Build history of the part. All positions in model axes, mm. A direction names the side the tool comes from. Give positions to 0.01 mm unless a question says otherwise; leave off trailing zeros. One line per item, written item: value.
```python
from build123d import *

# Parameters (mm, degrees)
F2_R     = 2.54
F3_R     = 1
F4_W     = 19.7092390154
F4_H     = 15.7092064619
F5_DEPTH = 22.4


with BuildPart() as f1:
    # F0 (on Front) → F1 (revolve)
    with BuildSketch(Plane.XZ):
        with BuildLine():
            Line((0, 130), (0, 0))
            Line((0, 0), (17.5, 0))
            add(Edge.make_bspline(
                [(17.5, 130), (22.5, 119.6596379665), (24.4853151406, 100.3614181833), (17.1932288242, 80.5399245506), (13.9866485718, 64.883493419), (17.1932288242, 49.9643932696), (24.4853151406, 27.3672993347), (22.5, 16.2580761236), (17.5, 0)],
                knots=[0, 0, 0, 0, 0.1975961429, 0.3602784274, 0.5, 0.6397215726, 0.8024038571, 1, 1, 1, 1], degree=3))
            add(Edge.make_bspline(
                [(3, 205), (1.2158900885, 130), (5.5774394423, 104.8566326499), (17.5, 130)],
                knots=[0, 0, 0, 0, 76.3888080808, 76.3888080808, 76.3888080808, 76.3888080808], degree=3))
            Line((3, 205), (0, 205))
            Line((0, 205), (0, 130))
        make_face()
        Polygon((0, 210), (0, 205), (3, 205), (5, 205), (5, 210), align=None)
    revolve(axis=Axis((0, 0, 65), (0, 0, 1)))

    # F2
    f2_edges = [f1.edges().sort_by_distance(p)[0] for p in [
        (-17.5, 0, 0),
    ]]
    fillet(f2_edges, radius=F2_R)

    # F3
    f3_edges = [f1.edges().sort_by_distance(p)[0] for p in [
        (-5, 0, 205),
        (-5, 0, 210),
    ]]
    fillet(f3_edges, radius=F3_R)

    # F4 (on Front) → F5 (cut, symmetric)
    with BuildSketch(Plane.XZ):
        with Locations((-13.3473322494, 209.7727283835)):
            Rectangle(F4_W, F4_H)
    extrude(amount=F5_DEPTH, both=True, mode=Mode.SUBTRACT)


solid = f1.part
```
(1) 3-axis set-ups, long thin cutter, end or side, ignore diameter. For faces 4 (the face through (-3.493, 0, 207)), 5 (the face through (5, 0, 208)): which of +Z, -Z, +X, -X, +Y, -Y reach the whole face in a straight line?
Completed:
face 4: +Z, -X, +Y, -Y
face 5: +Z
(2) Pin check, flat tips, straight feed: P1, Ø1.5, axis at y = 0, z = 207, coming from the -X side; P2, Ø8, axis at x = 10, z = 58, coming from the +Y side; P3, Ø5, axis at y = 14, z = 54.5, coming from the +X side. Stop position of each tip, or through.
Completed:
P1: x = -3.49
P2: y = 14.64
P3: x = 11.77
(3) Pull direction Z, two halves, no side cores. Call faces 1 (the face through (3, 1, 205)), 2 (the face through (0, 0, 0)), 3 (the face through (0, 0, 210)): +Z half, -Z half, draft (parallel to the pull), parting line (faces both ways), or undercut.
Completed:
face 1: undercut
face 2: -Z half
face 3: +Z half
(4) Drill centre lines: line 1 (X direction, y = 9, z = 128); line 2 (X direction, y = 9, z = 64); line 3 (X direction, y = 12.5, z = 17). Where is each one in solid material? Low to high.
Completed:
line 1: -16.07 to -13.84, 13.84 to 16.07
line 2: -12.02 to 12.02
line 3: -18.18 to 18.18
